Geometry: see drawing. Coordinates: mm, zero at the bounding-box minimum. A direction names the side the tool comes from. Give positions to 0.01 mm unless a question says otherwise; leave off trailing zeros. Write each loop counter-clockwise with the first axis right and the second up, starting at its lowest first coordinate (ties: lowest second). Pieces come first, ordered by that corner, then holes.
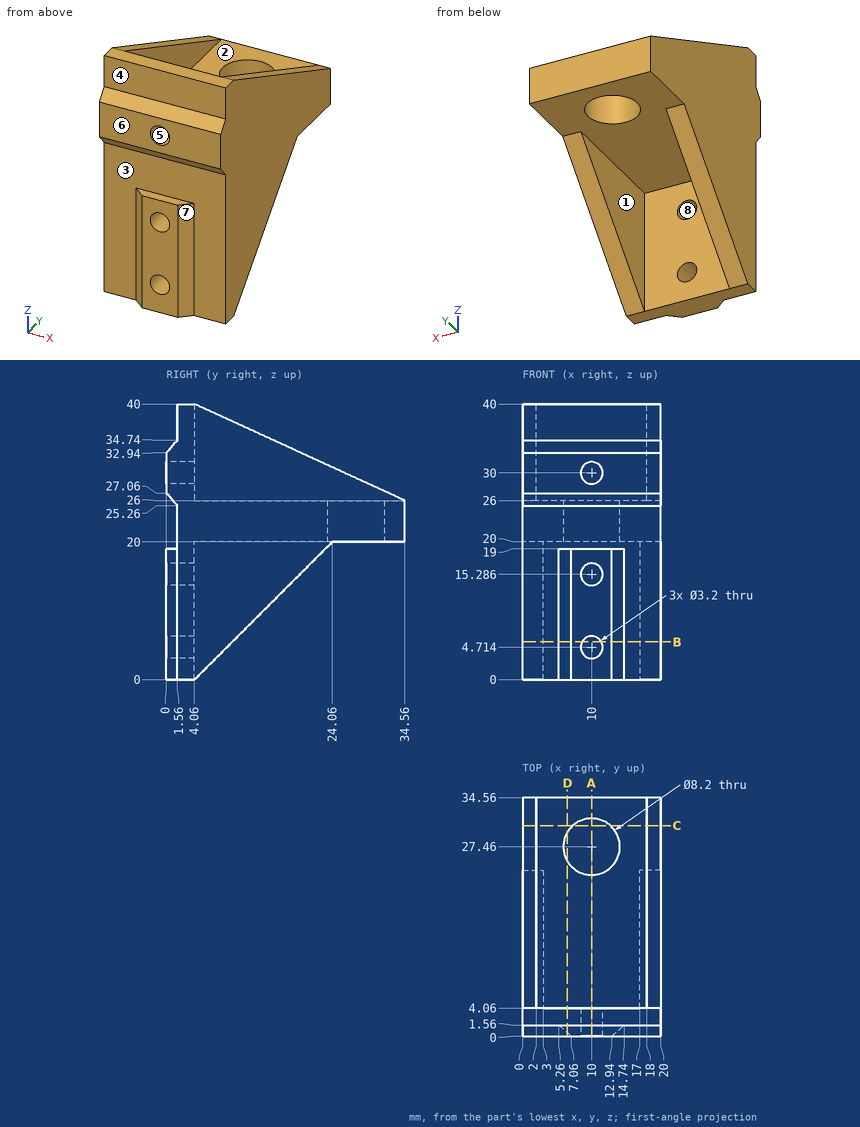
1. Line query: probe 1 along Z at (x, y) = (10, 3.2); probe 2 along Y at (x, z) = (10, 21.35); probe 3 along X at (y, z) = (8, 14). Output: solid intervals per line, ascending.
2. Section query B-B (z = 5.5). Return loops of the section in (x, y).
3. Section query C-C (y = 30.5). Return loops of the section in (x, z), plus the area to 3 significant figures.
4. Pull-direction query (X, two-part tool) for the marked faces 5, 6, 7 and 8; classes: pulls with the +X half, pulls with the -X half, needs draft (parallel to the pull), parting line crosses it, or undercut.
5. Pin query (flat end, axial travel): P1, Ø12, axis at x = 16.5, y = 24, coming from the -Z side; P2, Ø1.7, axis at x = 11, y = 0.5, coming from the +Z side; P3, Ø3, axis at x = 6.5, y = 7, coming from the -Z side; P4, Ø1.5, axis at y = 19, z = 36, coming from the +X side. Return the tip coordinate at first contact, or that it passes through.
6. Access query for the marked faces 1, 2, 3 and 4. Directions: +Z, -Z, +X, -X, +Y, -Y. A direction counts if a zero-diameter tool reaches every point of the face in a straight line with its end or side. Return the directions, or none.
7. Section query A-A (x = 10). Give the number of separate pieces and of enclosed holes in the cut face, plus the area to 3 significant figures.
8. Section query D-D (x = 6.5). Return loops of the section in (y, z).
The answers:
1. probe 1: z = 0 to 3.11, 6.31 to 13.69, 16.89 to 28.4, 31.6 to 40
1. probe 2: y = 1.56 to 23.36, 31.56 to 34.56
1. probe 3: x = 0 to 3, 17 to 20
2. outline: (0, 1.56) - (5.26, 1.56) - (7.06, 0) - (8.61, 0) - (8.61, 4.06) - (3, 4.06) - (3, 9.56) - (0, 9.56) - close; (11.39, 0) - (12.94, 0) - (14.74, 1.56) - (20, 1.56) - (20, 9.56) - (17, 9.56) - (17, 4.06) - (11.39, 4.06) - close
3. outline: (0, 20) - (7.25, 20) - (7.25, 26) - (2, 26) - (2, 27.86) - (0, 27.86) - close; (12.75, 20) - (20, 20) - (20, 27.86) - (18, 27.86) - (18, 26) - (12.75, 26) - close
3. area: 94.4 mm2
4. face 5: undercut
4. face 6: needs draft
4. face 7: pulls with the +X half
4. face 8: undercut
5. P1: stops at z = 13.96
5. P2: stops at z = 34.5
5. P3: stops at z = 20
5. P4: passes through
6. face 1: -Z, +Y
6. face 2: +Z, +Y
6. face 3: -Y
6. face 4: +Z, +X, -X, -Y
7. separate pieces: 5
7. enclosed holes: 0
7. area: 236 mm2
8. outline: (0, 27.06) - (1.56, 25.26) - (1.56, 19) - (0.49, 19) - (0.49, 0) - (4.06, 0) - (4.06, 20) - (25.32, 20) - (25.32, 26) - (4.06, 26) - (4.06, 40) - (1.56, 40) - (1.56, 34.74) - (0, 32.94) - close; (29.6, 20) - (34.56, 20) - (34.56, 26) - (29.6, 26) - close
